The listing builds one solid part. Answer for the finished solid, in the listing's coordinates (mm). Round coordinates to 2 decimals unless told otherwise and drop trailing zeros. Write each loop counter-clockwise with the first axis right and the second up, starting at its lowest first coordinate (ties: lowest second). Pieces come first, ordered by that corner, then holes. Notation, with made-up numbers: (82, -7.5) - (126, -7.5) arc R30 cw to (126, 14.5) - close; hole circle Ø9 at (-38, 61). An arc over 180 degrees is marked (long way). Return JSON: item names as keys, results as strings. Group by question number.
from build123d import *

# Parameters (mm, degrees)
F0_W     = 38.1
F0_H     = 19.05
F1_DEPTH = 9.525
F2_R     = 1.5875
F3_DEPTH = 9.525
F4_R     = 0.7874
F5_D     = 12.954


with BuildPart() as f1:
    # F0 (on Top) → F1 (new body)
    with BuildSketch(Plane.XY):
        Rectangle(F0_W, F0_H)
    extrude(amount=F1_DEPTH)

    # F2 (on face) → F3 (cut, through all)
    with BuildSketch(Plane.XY.offset(9.525)):
        with Locations((-14.986, 0)):
            Circle(F2_R)
        with Locations((14.986, 0)):
            Circle(F2_R)
    extrude(amount=-F3_DEPTH, mode=Mode.SUBTRACT)

    # F4
    f4_edges = [f1.edges().sort_by_distance(p)[0] for p in [
        (0, -9.525, 9.525),
        (-19.05, 0, 9.525),
        (0, 9.525, 9.525),
        (19.05, 0, 9.525),
        (19.05, -9.525, 4.7625),
        (19.05, 9.525, 4.7625),
        (-19.05, -9.525, 4.7625),
        (-19.05, 9.525, 4.7625),
    ]]
    fillet(f4_edges, radius=F4_R)

    # F5 (through all)
    with Locations(Plane.XY.offset(9.525)):
        with Locations((0, 0)):
            Hole(F5_D / 2)


solid = f1.part
(1) Determine the mould class of faces 1 (the flat face through (-4, 6, 9.525)), 2 (the cylindrical face through (-16.57, 0.07, 4.83)), 3 (the flat face through (19.05, 0, 4)) for opening direction X: +X half, -X half, draft (parallel to the pull), parting line (faces both ways), or undercut.
(2) Flat-ended cylindrical pins translate along their axes: pin 1 (10 mm diameter, centred on x = 12.5, y = -6, fed in from -Z); pin 2 (1.9 mm diameter, centred on x = -14.986, y = 0, fed in from +Z). Find the tip coordinate at first contact, or state that the pin passes through.
(3) Find section B-B (x = 0). Write down the section's boundary in (y, z) (3 decimals), plus the area to 3 significant figures.
(4) Find section D-D (x = 15). Write down the section's boundary in (y, z) (3 decimals).
(5) Find section A-A (y = 0). State how many separate pieces and enclosed holes the cut face has, plus the area to 3 significant figures.
(6) Consider line 1 (X direction, y = -0.5, z = 8.25); line 2 (X direction, y = -1, z = 3.75); line 3 (Y direction, x = 5, z = 4) (3 decimals). Determine where each line is inside the solid, lowest interval first.
Check sheet entries:
{
 "1": {"face 1": "draft", "face 2": "undercut", "face 3": "+X half"},
 "2": {"pin 1": "stops at z = 0", "pin 2": "passes through"},
 "3": {"outline": "(-9.525, 0) - (-6.477, 0) - (-6.477, 9.525) - (-8.738, 9.525) arc R0.787 ccw to (-9.525, 8.738) - close; (6.477, 0) - (9.525, 0) - (9.525, 8.738) arc R0.787 ccw to (8.738, 9.525) - (6.477, 9.525) - close", "area": "57.8 mm^2"},
 "4": {"outline": "(-9.525, 0) - (-1.587, 0) - (-1.587, 9.525) - (-8.738, 9.525) arc R0.787 ccw to (-9.525, 8.738) - close; (1.587, 0) - (9.525, 0) - (9.525, 8.738) arc R0.787 ccw to (8.738, 9.525) - (1.587, 9.525) - close"},
 "5": {"separate pieces": "4", "enclosed holes": "0", "area": "179 mm^2"},
 "6": {"line 1": "x = -19.05 to -16.49, -13.48 to -6.46, 6.46 to 13.48, 16.49 to 19.05", "line 2": "x = -19.05 to -16.22, -13.75 to -6.4, 6.4 to 13.75, 16.22 to 19.05", "line 3": "y = -9.525 to -4.117, 4.117 to 9.525"}
}
